Could you check a few things on this model? Use its own coordinates, in mm. Face numbers are marked on the shaded views. A direction names the side the tool comes from. Round coordinates to 2 decimals unless told otherwise and drop trailing zeros. Write each loop counter-clockwise with the first axis right and the second up, starting at its lowest first coordinate (ties: lowest second). Pieces come first, ordered by that corner, then holes. Notation, with made-up numbers: (-36.5, 19.25) - (-11.5, 19.25) arc R19 ccw to (-11.5, 51.25) - close; hole circle Ø6 at (60.25, 8.5). An arc over 180 degrees is marked (long way). Put each result on its own line as item: value.
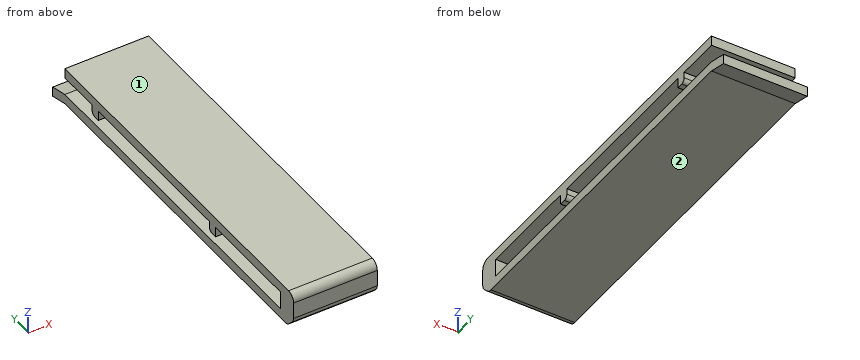
from build123d import *

# Parameters (mm, degrees)
F0_W     = 2.694248
F0_H     = 4.5
F0_H_2   = 2.5
F0_W_2   = 86.305752
F0_W_3   = 26
F0_W_4   = 2.5
F1_DEPTH = 21
F2_R     = 2
F3_R     = 1


with BuildPart() as f1:
    # F0 (on Right) → F1 (new body)
    with BuildSketch(Plane.YZ):
        Polygon((23.180372, 8.721056), (23.180372, 6.221056), (67.568183, 6.221056), (70.068183, 6.221056), (80.986124, 6.221056), (80.986124, 8.721056), align=None)
        with Locations((-6.666752, 3.971056)):
            Rectangle(F0_W, F0_H)
        with Locations((-6.666752, 0.471056)):
            Rectangle(F0_W, F0_H_2)
        with Locations((37.833248, 0.471056)):
            Rectangle(F0_W_2, F0_H_2)
        with Locations((7.680372, 7.471056)):
            Rectangle(F0_W_3, F0_H_2)
        Polygon((-8.013876, -0.778944), (-8.013876, 1.721056), (-8.013876, 6.221056), (-8.013876, 8.721056), (-10.4775, 8.721056), (-10.4775, 7.235875), (-10.4775, 1.721056), align=None)
        with Locations((-6.666752, 7.471056)):
            Rectangle(F0_W, F0_H_2)
        with Locations((21.930372, 7.471056)):
            Rectangle(F0_W_4, F0_H_2)
        with Locations((68.818183, 4.971056)):
            Rectangle(F0_W_4, F0_H_2)
        with Locations((21.930372, 4.971056)):
            Rectangle(F0_W_4, F0_H_2)
        Polygon((85.827354, 0.471056), (80.986124, 1.721056), (80.986124, -0.778944), (85.827354, -2.028944), align=None)
    extrude(amount=F1_DEPTH)

    # F2
    f2_edges = [f1.edges().sort_by_distance(p)[0] for p in [
        (10.5, -10.4775, 8.721056),
        (10.5, -8.013876, -0.778944),
        (10.5, -10.4775, 1.721056),
    ]]
    fillet(f2_edges, radius=F2_R)

    # F3
    f3_edges = [f1.edges().sort_by_distance(p)[0] for p in [
        (10.5, 23.180372, 3.721056),
        (10.5, 70.068183, 3.721056),
    ]]
    fillet(f3_edges, radius=F3_R)


solid = f1.part
(1) For the marked faces 1 and 2, which set-ups out of +Z, -Z, +X, -X, +Y, -Y let a thin tool reach every point of the face, with its end or its side?
Values found:
face 1: +Z, +X, -X, +Y, -Y
face 2: -Z, +X, -X, -Y
(2) Please list where these lines run through material, in increasing order: probe 1 along Y at (x, z) = (4.75, 6); probe 2 along Z at (x, y) = (2.25, 35); probe 3 along Z at (x, y) = (20, 22). Write a range as from..to.
Values found:
probe 1: y = -10.48..-5.32, 20.68..23.18, 67.57..70.07
probe 2: z = -0.78..1.72, 6.22..8.72
probe 3: z = -0.78..1.72, 3.72..8.72
(3) Imagine slicing it at A-A, the plane y = 49.5. List the corners of the cut face in (x, z) for me, then the cut area to 3 significant figures.
Values found:
outline: (0, -0.78) - (21, -0.78) - (21, 1.72) - (0, 1.72) - close; (0, 6.22) - (21, 6.22) - (21, 8.72) - (0, 8.72) - close
area: 105 mm^2
(4) Imagine slicing it at B-B, the plane x = 3.75. List the corners of the cut face in (y, z) for me.
Values found:
outline: (-10.48, 2.54) arc R2 ccw to (-9.9, 1.14) - (-8.6, -0.18) arc R2 ccw to (-7.18, -0.78) - (80.99, -0.78) - (85.83, -2.03) - (85.83, 0.47) - (80.99, 1.72) - (-5.32, 1.72) - (-5.32, 6.22) - (20.68, 6.22) - (20.68, 3.72) - (22.18, 3.72) arc R1 ccw to (23.18, 4.72) - (23.18, 6.22) - (67.57, 6.22) - (67.57, 3.72) - (69.07, 3.72) arc R1 ccw to (70.07, 4.72) - (70.07, 6.22) - (80.99, 6.22) - (80.99, 8.72) - (-8.48, 8.72) arc R2 ccw to (-10.48, 6.72) - close
(5) I'm going to push flat-ended pins straight in: pin 1 (6 mm diameter, centred on x = 18, y = 62.5, fed in from -Z); pin 2 (12 mm diameter, centred on x = 9, y = 77.5, fed in from -Z); pin 3 (1.5 mm diameter, centred on y = 63, z = 5, fed in from +X); pin 4 (2 mm diameter, centred on x = 14.5, z = 7, fed in from +Y). Where does each tip first touch, or does it pass through?
Values found:
pin 1: stops at z = -0.78
pin 2: stops at z = -1.43
pin 3: passes through
pin 4: stops at y = 80.99
